```python
from build123d import *

# Parameters (mm, degrees)
BOSS_EXTRUDE1_DEPTH       = 9.525
F_6_0MM_DOWEL_HOLE1_D     = 6.1
SKETCH4_R                 = 31.5
CUT_EXTRUDE1_DEPTH        = 68.847075287
F_4_0MM_DOWEL_HOLE1_D     = 4
F_4_0MM_DOWEL_HOLE1_DEPTH = 3.2
F_4_0MM_DOWEL_HOLE1_TIP   = 1.201721238
F_4_0MM_DOWEL_HOLE2_D     = 4
F_4_0MM_DOWEL_HOLE2_DEPTH = 3.2
F_4_0MM_DOWEL_HOLE2_TIP   = 1.201721238


with BuildPart() as part:
    # Sketch1 → Boss-Extrude1 (new body)
    with BuildSketch(Plane.XY):
        with BuildLine():
            Line((-25, 47.5), (25, 47.5))
            Line((25, 47.5), (39.154013015, 26.892624729))
            ThreePointArc((39.154013015, 26.892624729), (47.5, 0), (39.154013015, -26.892624729))
            Line((39.154013015, -26.892624729), (25, -47.5))
            Line((25, -47.5), (-25, -47.5))
            Line((-25, -47.5), (-39.154013015, -26.892624729))
            ThreePointArc((-39.154013015, -26.892624729), (-47.5, 0), (-39.154013015, 26.892624729))
            Line((-39.154013015, 26.892624729), (-25, 47.5))
        make_face()
    extrude(amount=-BOSS_EXTRUDE1_DEPTH)

    # Ø6.0mm Dowel Hole1 (through all)
    with Locations(Plane.XY):
        with Locations((-30.743901834, 17.75), (0, 35.5), (30.743901834, 17.75), (30.743901834, -17.75), (0, -35.5), (-30.743901834, -17.75)):
            Hole(F_6_0MM_DOWEL_HOLE1_D / 2)

    # Sketch4 → Cut-Extrude1 (cut, through all)
    with BuildSketch(Plane(origin=(0, 0, -9.525), x_dir=(-1, 0, 0), z_dir=(0, 0, -1))):
        Circle(SKETCH4_R)
    extrude(amount=-CUT_EXTRUDE1_DEPTH, mode=Mode.SUBTRACT)

    # Ø4.0mm Dowel Hole1
    with Locations(Plane(origin=(0, 47.5, 0), x_dir=(1, 0, 0), z_dir=(0, 1, 0))):
        with Locations((-16.67, 4.7625), (0, 4.7625), (16.67, 4.7625)):
            Hole(F_4_0MM_DOWEL_HOLE1_D / 2, depth=F_4_0MM_DOWEL_HOLE1_DEPTH)
            with Locations((0, 0, -(F_4_0MM_DOWEL_HOLE1_DEPTH + F_4_0MM_DOWEL_HOLE1_TIP / 2))):  # 118° drill point
                Cone(0, F_4_0MM_DOWEL_HOLE1_D / 2, F_4_0MM_DOWEL_HOLE1_TIP, mode=Mode.SUBTRACT)

    # Ø4.0mm Dowel Hole2
    with Locations(Plane.XZ.offset(47.5)):
        with Locations((0, -4.7625), (-16.67, -4.7625), (16.67, -4.7625)):
            Hole(F_4_0MM_DOWEL_HOLE2_D / 2, depth=F_4_0MM_DOWEL_HOLE2_DEPTH)
            with Locations((0, 0, -(F_4_0MM_DOWEL_HOLE2_DEPTH + F_4_0MM_DOWEL_HOLE2_TIP / 2))):  # 118° drill point
                Cone(0, F_4_0MM_DOWEL_HOLE2_D / 2, F_4_0MM_DOWEL_HOLE2_TIP, mode=Mode.SUBTRACT)


solid = part.part
```
CAD build for the part. Positions are in the model's coordinates, mm. A direction names the side the tool comes from. Round coordinates to 2 decimals unless told otherwise and drop trailing zeros. Order: outer loops, then holes, each group sorted by start corner. A loop starts at its lowest first (then second) coordinate and runs counter-clockwise, first axis right, second up.
Q1. Two-plate mould, pull along X, no slides. Class faces 1 (the conical face through (-16.349, -43.307, -4.896)), 2 (the flat face through (0, -47.5, -7)), 3 (the flat face through (-31.98, -37.34, -4.7)), 4 (the flat face through (31.98, 37.34, -4.7)): pulls with the +X half, pulls with the -X half, needs draft (parallel to the pull), parting line crosses it, or undercut.
Q2. Drop flat-ended pins along their axis: pin 1 (1 mm diameter, centred on y = 11, z = -5, fed in from -X); pin 2 (3 mm diameter, centred on x = 16.67, z = -4.76, fed in from +Y); pin 3 (2.5 mm diameter, centred on x = 16.67, z = -4.76, fed in from +Y); pin 4 (7 mm diameter, centred on x = 0, y = 35.5, fed in from -Z) (3 decimals). Give the stop position or say it passes through.
Q3. Slice it at D-D (x = -35). Write the cut outline in (y, z) (3 decimals).
Q4. Slice it at A-A (z = -8). Write the cut outline in (x, y).
Q5. Which spindle directions (+Z, -Z, +X, -X, +Y, -Y) get a long thin tool onto all of the face, cutting with end or side? Do faces 5 (the cylindrical face through (18.257, -45.878, -5.979)), 6 (the cylindrical face through (4.101, 31.232, -4.829)), 7 (the cylindrical face through (-18.58, 45.88, -5.36)). Say none if no direction does.
Q6. Slice it at C-C (y = 22). Write the cut outline in (x, z) (3 decimals).
Q7. Slice it at B-B (y = -10.5). Write the cut outline in (x, z) (3 decimals).
Q8. Wall check: L1, parallel to Y at x = 0, z = -7.5; L2, parallel to Y at x = -15, z = -8.5; L3, parallel to Y at x = 29, z = -1.5. Give the ranges that are in metal, low to high.
Results below:
1. face 1: undercut
1. face 2: needs draft
1. face 3: pulls with the -X half
1. face 4: pulls with the +X half
2. pin 1: stops at x = -46.32
2. pin 2: stops at y = 44
2. pin 3: stops at y = 43.85
2. pin 4: stops at z = -9.525
3. outline: (-32.941, -9.525) - (32.941, -9.525) - (32.941, 0) - (-32.941, 0) - close
4. outline: (-39.15, -26.89) - (-25, -47.5) - (25, -47.5) - (39.15, -26.89) arc R47.5 ccw to (39.15, 26.89) - (25, 47.5) - (-25, 47.5) - (-39.15, 26.89) arc R47.5 ccw to start; hole circle Ø6.1 at (-30.74, -17.75); hole circle Ø6.1 at (-30.74, 17.75); hole circle Ø63 at (0, 0); hole circle Ø6.1 at (0, -35.5); hole circle Ø6.1 at (0, 35.5); hole circle Ø6.1 at (30.74, -17.75); hole circle Ø6.1 at (30.74, 17.75)
5. face 5: -Y
5. face 6: +Z, -Z
5. face 7: +Y
6. outline: (-42.098, -9.525) - (-22.544, -9.525) - (-22.544, 0) - (-42.098, 0) - close; (22.544, -9.525) - (42.098, -9.525) - (42.098, 0) - (22.544, 0) - close
7. outline: (-46.325, -9.525) - (-29.698, -9.525) - (-29.698, 0) - (-46.325, 0) - close; (29.698, -9.525) - (46.325, -9.525) - (46.325, 0) - (29.698, 0) - close
8. L1: y = -47.5 to -38.55, -32.45 to -31.5, 31.5 to 32.45, 38.55 to 47.5
8. L2: y = -47.5 to -27.7, 27.7 to 47.5
8. L3: y = -41.68 to -20.25, -15.25 to -12.3, 12.3 to 15.25, 20.25 to 41.68
